```python
from build123d import *

# Parameters (mm, degrees)
SKETCH1_R           = 9
BOSS_EXTRUDE1_DEPTH = 18.4
SKETCH2_R           = 10.75
BOSS_EXTRUDE2_DEPTH = 2.6
SKETCH3_R           = 7.75
CUT_EXTRUDE1_DEPTH  = 3
SKETCH4_R           = 9
SKETCH4_R_2         = 8
CUT_EXTRUDE2_DEPTH  = 10
CUT_EXTRUDE3_DEPTH  = 8.4
CUT_EXTRUDE4_DEPTH  = 19.4
FILLET1_R           = 0.5


with BuildPart() as part:
    # Sketch1 → Boss-Extrude1 (new body)
    with BuildSketch(Plane.XY):
        Circle(SKETCH1_R)
    extrude(amount=-BOSS_EXTRUDE1_DEPTH)

    # Sketch2 → Boss-Extrude2 (add)
    with BuildSketch(Plane.XY):
        Circle(SKETCH2_R)
    extrude(amount=BOSS_EXTRUDE2_DEPTH)

    # Sketch3 → Cut-Extrude1 (cut)
    with BuildSketch(Plane.XY.offset(2.6)):
        Circle(SKETCH3_R)
    extrude(amount=-CUT_EXTRUDE1_DEPTH, mode=Mode.SUBTRACT)

    # Sketch4 → Cut-Extrude2 (cut)
    with BuildSketch(Plane(origin=(0, 0, -18.4), x_dir=(-1, 0, 0), z_dir=(0, 0, -1))):
        Circle(SKETCH4_R)
        Circle(SKETCH4_R_2, mode=Mode.SUBTRACT)
    extrude(amount=-CUT_EXTRUDE2_DEPTH, mode=Mode.SUBTRACT)

    # Sketch5 → Cut-Extrude3 (cut)
    with BuildSketch(Plane(origin=(0, 0, -8.4), x_dir=(-1, 0, 0), z_dir=(0, 0, -1))):
        with BuildLine():
            Line((-8.5, 2.958039892), (-8.5, -2.958039892))
            ThreePointArc((-8.5, -2.958039892), (-9, 0), (-8.5, 2.958039892))
        make_face()
        with BuildLine():
            Line((8.5, 2.958039892), (8.5, -2.958039892))
            ThreePointArc((8.5, -2.958039892), (9, 0), (8.5, 2.958039892))
        make_face()
        with BuildLine():
            ThreePointArc((-1.636306817, 8.85), (0, 8), (1.636306817, 8.85))
            ThreePointArc((1.636306817, 8.85), (0, 9), (-1.636306817, 8.85))
        make_face()
    extrude(amount=-CUT_EXTRUDE3_DEPTH, mode=Mode.SUBTRACT)

    # Sketch6 → Cut-Extrude4 (cut, through all)
    with BuildSketch(Plane.XY):
        with BuildLine():
            Line((-3.25, 1.625), (3.25, 1.625))
            ThreePointArc((3.25, 1.625), (4.133883476, 1.258883476), (4.5, 0.375))
            Line((4.5, 0.375), (4.5, -0.375))
            ThreePointArc((4.5, -0.375), (4.133883476, -1.258883476), (3.25, -1.625))
            Line((3.25, -1.625), (-3.25, -1.625))
            ThreePointArc((-3.25, -1.625), (-4.133883476, -1.258883476), (-4.5, -0.375))
            Line((-4.5, -0.375), (-4.5, 0.375))
            ThreePointArc((-4.5, 0.375), (-4.133883476, 1.258883476), (-3.25, 1.625))
        make_face()
    extrude(amount=-CUT_EXTRUDE4_DEPTH, mode=Mode.SUBTRACT)

    # Fillet1
    fillet1_edges = [part.edges().sort_by_distance(p)[0] for p in [
        (-7.75, 0, -0.4),
        (-4.133883476, 1.258883476, -0.4),
        (0, 1.625, -0.4),
        (4.133883476, 1.258883476, -0.4),
        (4.5, 0, -0.4),
        (4.133883476, -1.258883476, -0.4),
        (0, -1.625, -0.4),
        (-4.133883476, -1.258883476, -0.4),
        (-4.5, 0, -0.4),
        (-10.75, 0, 2.6),
    ]]
    fillet(fillet1_edges, radius=FILLET1_R)


solid = part.part
```
The listing builds one solid part. Answer for the finished solid, in the listing's coordinates (mm). A direction names the side the tool comes from. Coordinates: 2 decimals unless noted, no trailing zeros. Loops run counter-clockwise (first coordinate to the right, second up) from the corner with the lowest first, then second, coordinate; pieces in that order, holes last. Notation, with made-up numbers: (30, 66.5) - (42, 66.5) arc R4 ccw to (42, 70.5) - close; hole circle Ø11 at (71, 20). An arc over 180 degrees is marked (long way). Write item = value, one per line.
1) Find the intervals of material crossed by line 1 along Y through (x, z) = (0, 2.05); line 2 along X through (y, z) = (2.25, -2.75); line 3 along Z through (x, y) = (2, -9.5), in increasing order.
Responses:
line_1 = -10.75 to -7.75, 7.75 to 10.75
line_2 = -8.5 to 8.5
line_3 = 0 to 2.6
2) Section A-A (y = 0) is taken. Determine the outline of the cut face in (x, z), plus the area to 3 significant figures.
Responses:
outline = (-10.75, 0) - (-8.5, 0) - (-8.5, -8.4) - (-8, -8.4) - (-8, -18.4) - (-4.5, -18.4) - (-4.5, -0.9) arc R0.5 ccw to (-5, -0.4) - (-7.25, -0.4) arc R0.5 cw to (-7.75, 0.1) - (-7.75, 2.6) - (-10.25, 2.6) arc R0.5 ccw to (-10.75, 2.1) - close; (4.5, -18.4) - (8, -18.4) - (8, -8.4) - (8.5, -8.4) - (8.5, 0) - (10.75, 0) - (10.75, 2.1) arc R0.5 ccw to (10.25, 2.6) - (7.75, 2.6) - (7.75, 0.1) arc R0.5 cw to (7.25, -0.4) - (5, -0.4) arc R0.5 ccw to (4.5, -0.9) - close
area = 150 mm^2
3) Section C-C (z = -11.25) is taken. Determine the outline of the cut face in (x, y) (3 decimals), plus the area to 3 significant figures.
Responses:
outline = circle Ø16 at (0, 0); hole (-4.5, -0.375) arc R1.25 ccw to (-3.25, -1.625) - (3.25, -1.625) arc R1.25 ccw to (4.5, -0.375) - (4.5, 0.375) arc R1.25 ccw to (3.25, 1.625) - (-3.25, 1.625) arc R1.25 ccw to (-4.5, 0.375) - close
area = 173 mm^2
4) Each of these flat-tipped pins is pushed along its axis until it touches: P1, Ø3, axis at x = 0, z = -11, coming from the -Y side; P2, Ø4.5, axis at y = -0.5, z = -5.5, coming from the +X side; P3, Ø4, axis at y = -3.5, z = -0.5, coming from the -X side; P4, Ø5, axis at x = 7, y = 5.5, coming from the -Z side. Where does it stop, or does it pass through?
Responses:
P1 = -8
P2 = 8.5
P3 = -10.64
P4 = -18.4
5) Section B-B (z = -4) is taken. Determine the outline of the cut face in (x, y) (3 decimals).
Responses:
outline = (-8.5, -2.958) arc R9 ccw to (8.5, -2.958) - (8.5, 2.958) arc R9 ccw to (1.636, 8.85) arc R2 cw to (-1.636, 8.85) arc R9 ccw to (-8.5, 2.958) - close; hole (-4.5, -0.375) arc R1.25 ccw to (-3.25, -1.625) - (3.25, -1.625) arc R1.25 ccw to (4.5, -0.375) - (4.5, 0.375) arc R1.25 ccw to (3.25, 1.625) - (-3.25, 1.625) arc R1.25 ccw to (-4.5, 0.375) - close
6) Which of the six approach directions +Z, -Z, +X, -X, +Y, -Y give full straight-line access (tool end or side, diameter ignored) to faces 5 (the face through (-8.5, 0, -4)), 6 (the face through (8.5, 0, -4)), 7 (the face through (0, -1.625, -10)), 8 (the face through (5.91, 6.79, -4.14))?
Responses:
face_5 = -Z, -X, +Y, -Y
face_6 = -Z, +X, +Y, -Y
face_7 = +Z, -Z
face_8 = -Z, +X, +Y
7) Determine the mould class of faces 1 (the face through (-5.812, 6.872, -4.141)), 2 (the face through (0, -3, -0.4)), 3 (the face through (2, -8, -8.4)), 4 (the face through (4.14, -1.25, -9.53)) for opening direction X: pulls with the +X half, pulls with the -X half, needs draft (parallel to the pull), parting line crosses it, or undercut.
Responses:
face_1 = pulls with the -X half
face_2 = undercut
face_3 = needs draft
face_4 = undercut
